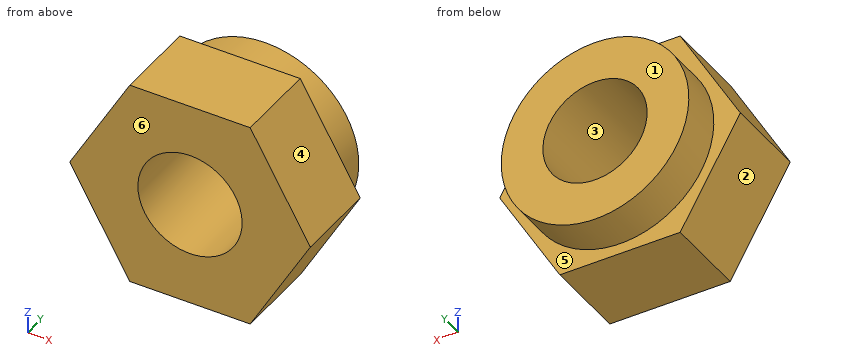
from build123d import *

# Parameters (mm, degrees)
EXTRUDE_1_DEPTH     = 3
CUT_EXTRUDE_1_REACH = 6.856
SKETCH_2_R          = 1.25
SKETCH_3_OUTSIDE_W  = 9.416
SKETCH_3_OUTSIDE_H  = 8.642
SKETCH_3_OUTSIDE_R  = 2.25
CUT_EXTRUDE_2_DEPTH = 1


with BuildPart() as part:
    # 草图1 → 凸台-拉伸1 (new body)
    with BuildSketch(Plane(origin=(0, 0, 0), x_dir=(1, 0, 0), z_dir=(0, 1, 0))):
        Polygon((2.886751346, 0), (1.443375673, 2.5), (-1.443375673, 2.5), (-2.886751346, 0), (-1.443375673, -2.5), (1.443375673, -2.5), align=None)
    extrude(amount=EXTRUDE_1_DEPTH)

    # 草图2 → 切除-拉伸1 (cut, up to next)
    with BuildSketch(Plane(origin=(0, 3, 0), x_dir=(1, 0, 0), z_dir=(0, 1, 0)), mode=Mode.PRIVATE) as cut_extrude_1_sk1:
        with Locations(Location((0, 0, 0), (0, 0, 270))):
            Circle(SKETCH_2_R)
    cut_extrude_1_tool1 = extrude(cut_extrude_1_sk1.sketch, amount=-CUT_EXTRUDE_1_REACH, mode=Mode.PRIVATE) & part.part
    add(cut_extrude_1_tool1.solids().sort_by_distance((0, 3, 0))[0], mode=Mode.SUBTRACT)

    # 草图3 outside → 切除-拉伸2 (cut)
    with BuildSketch(Plane(origin=(0, 3, 0), x_dir=(1, 0, 0), z_dir=(0, 1, 0))):
        Rectangle(SKETCH_3_OUTSIDE_W, SKETCH_3_OUTSIDE_H)
        with Locations(Location((0, 0, 0), (0, 0, 270))):
            Circle(SKETCH_3_OUTSIDE_R, mode=Mode.SUBTRACT)
    extrude(amount=-CUT_EXTRUDE_2_DEPTH, mode=Mode.SUBTRACT)


solid = part.part
CAD build for the part. Positions are in the model's coordinates, mm. Face numbers are marked on the shaded views. A direction names the side the tool comes from. Coordinates: 2 decimals unless noted, no trailing zeros. Loops run counter-clockwise (first coordinate to the right, second up) from the corner with the lowest first, then second, coordinate; pieces in that order, holes last. Notation, with made-up numbers: (86, 39.5) - (107, 39.5) arc R25 ccw to (107, 51.5) - close; hole circle Ø7 at (69, 38). An arc over 180 degrees is marked (long way). Use one line per item in the form item = value. Start each with the question number.
1) Band-saw the part on A-A (y = 1.65). Give the cut face in (x, z).
2) Drill centre lines: L1, parallel to Z at x = 0.05, y = 0.3; L2, parallel to Y at x = 0.9, z = 2.15; L3, parallel to Z at x = -0.95, y = 2.1. Where is each one in solid material? Low to high. Write a range as from..to.
3) Flat gauge pin, fed straight in: pin 1 (2.5 mm diameter, centred on x = 0.5, z = -1, fed in from +Y). Where does the tip first touch, or does it go through?
4) Tool access for the marked faces 5 and 6: list every direction of +Z, -Z, +X, -X, +Y, -Y with a clear straight run to the whole face (end or side of a thin tool).
5) Two-plate mould, pull along Z, no slides. Class the marked faces 1, 2, 3 and 4: +Z half, -Z half, draft (parallel to the pull), parting line (faces both ways), or undercut.
6) Band-saw the part on D-D (z = -1.75). Give the cut face in (x, y).
7) Band-saw the part on C-C (z = 0.6). Give the cut face in (x, y), and give its area (3 significant figures).
8) Band-saw the part on B-B (x = 0). Give the cut face in (y, z).
Check values:
q1.outline = (-2.89, 0) - (-1.44, -2.5) - (1.44, -2.5) - (2.89, 0) - (1.44, 2.5) - (-1.44, 2.5) - close; hole circle Ø2.5 at (0, 0)
q2.L1 = -2.5..-1.25, 1.25..2.5
q2.L2 = 0..2
q2.L3 = -2.04..-0.81, 0.81..2.04
q3.pin_1 = 3
q4.face_5 = +Y
q4.face_6 = +Z, -Z, +X, -X, -Y
q5.face_1 = draft
q5.face_2 = -Z half
q5.face_3 = undercut
q5.face_4 = +Z half
q6.outline = (-1.88, 0) - (1.88, 0) - (1.88, 2) - (1.41, 2) - (1.41, 3) - (-1.41, 3) - (-1.41, 2) - (-1.88, 2) - close
q7.outline = (-2.54, 0) - (-1.1, 0) - (-1.1, 3) - (-2.17, 3) - (-2.17, 2) - (-2.54, 2) - close; (1.1, 0) - (2.54, 0) - (2.54, 2) - (2.17, 2) - (2.17, 3) - (1.1, 3) - close
q7.area = 7.92 mm2
q8.outline = (0, -2.5) - (2, -2.5) - (2, -2.25) - (3, -2.25) - (3, -1.25) - (0, -1.25) - close; (0, 1.25) - (3, 1.25) - (3, 2.25) - (2, 2.25) - (2, 2.5) - (0, 2.5) - close
